Check sheet for the modelled part. Datum: model origin and axes. Units: mm. A direction names the side the tool comes from. Coordinates: 2 decimals unless noted, no trailing zeros. Write each loop counter-clockwise with the first axis right and the second up, starting at its lowest first coordinate (ties: lowest second). Pieces come first, ordered by that corner, then holes. Notation, with made-up numbers: (6.5, -5) -> (40.5, -5) arc R17 cw to (40.5, 2) -> close; hole circle Ø2 at (-39.5, -38.5). An arc over 180 degrees is marked (long way). Put each result on its own line as item: value.
```python
from build123d import *

# Parameters (mm, degrees)
AUFSATZ_LINEAR_AUSTRAGEN1_DEPTH = 18
AUFSATZ_LINEAR_AUSTRAGEN2_DEPTH = 2
SCHNITT_LINEAR_AUSTRAGEN1_REACH = 31.142
SCHNITT_LINEAR_AUSTRAGEN2_REACH = 35.939
SKIZZE5_W                       = 12
SKIZZE5_H                       = 15
SKIZZE7_R                       = 1.22999984
AUFSATZ_LINEAR_AUSTRAGEN3_DEPTH = 6.5
SKIZZE8_R                       = 4.22999984
SKIZZE8_R_2                     = 2.3
AUFSATZ_LINEAR_AUSTRAGEN4_DEPTH = 3
SKIZZE9_W                       = 16.252283896
SKIZZE9_H                       = 8
SKIZZE9_W_2                     = 16.225392475
AUFSATZ_LINEAR_AUSTRAGEN7_DEPTH = 3
SCHNITT_LINEAR_AUSTRAGEN3_REACH = 3.5
SKIZZE11_W                      = 10
SKIZZE11_H                      = 10
SCHNITT_LINEAR_AUSTRAGEN4_REACH = 24.734
SKIZZE13_W                      = 10
SKIZZE13_H                      = 10
SCHNITT_LINEAR_AUSTRAGEN5_REACH = 24.815
SKIZZE14_W                      = 10
SKIZZE14_H                      = 10
SCHNITT_LINEAR_AUSTRAGEN6_REACH = 3.5
SKIZZE15_W                      = 10
SKIZZE15_H                      = 10
SCHNITT_LINEAR_AUSTRAGEN7_REACH = 24.918
SKIZZE16_W                      = 10
SKIZZE16_H                      = 10
SCHNITT_LINEAR_AUSTRAGEN8_REACH = 24.774
SKIZZE17_W                      = 10
SKIZZE17_H                      = 10


with BuildPart() as part:
    # Skizze1 → Aufsatz-Linear austragen1 (new body)
    with BuildSketch(Plane.XY):
        Polygon((-22.149859894, 27.765281808), (-11.635793215, 33.83000044), (-10.65000108, 33.83000044), (-10.65000108, 70.94999986), (10.5900012, 70.94999986), (10.5900012, 33.83000044), (11.612735063, 33.83000044), (21.946878227, 27.90320319), (54.822266278, 46.860690996), (65.431940836, 28.488460753), (35.875483821, 11.41999954), (37.79000014, 11.41999954), (37.79000014, -11.66999904), (36.372671479, -11.66999904), (65.402118422, -28.428154068), (54.791716349, -46.801638497), (21.961456264, -27.849347945), (11.636228403, -33.81000048), (10.608764603, -33.81000048), (10.588764643, -70.99999976), (-10.63000112, -70.99999976), (-10.63000112, -33.81000048), (-11.635211495, -33.81000048), (-21.94526311, -27.869445957), (-54.832668225, -46.841377939), (-65.441180026, -28.458395245), (-33.1799992, -9.82193495), (-33.1799992, 9.582671858), (-65.619428736, 28.349034811), (-55.023633975, 46.732102334), align=None)
        Polygon((-22.149950537, 26.033576659), (-11.234189479, 32.33000044), (-9.15000108, 32.33000044), (-9.15000108, 69.44999986), (9.0900012, 69.44999986), (9.0900012, 32.33000044), (11.2131258, 32.33000044), (21.948913697, 26.172853479), (54.272963006, 44.812413555), (63.382848908, 29.03729054), (31.311020441, 10.516235735), (31.653238716, 9.91999954), (36.29000014, 9.91999954), (36.29000014, -10.16999904), (31.252050971, -10.16999904), (31.132619329, -10.37701429), (63.352910716, -28.977183946), (54.242770108, -44.752743199), (21.961450411, -26.11734559), (11.234340849, -32.31000048), (9.109571053, -32.31000048), (9.089571093, -69.49999976), (-9.13000112, -69.49999976), (-9.13000112, -32.31000048), (-11.233987142, -32.31000048), (-21.945708018, -26.138007916), (-54.2831028, -44.792652518), (-63.392584266, -29.007267794), (-31.162137007, -10.388561496), (-31.6799992, -9.546253935), (-31.6799992, 9.963511331), (-31.471105622, 10.326986156), (-63.571974887, 28.897490395), (-54.473438465, 44.682904625), align=None, mode=Mode.SUBTRACT)
    extrude(amount=AUFSATZ_LINEAR_AUSTRAGEN1_DEPTH)

    # Skizze3 → Aufsatz-Linear austragen2 (add)
    with BuildSketch(Plane(origin=(0, 0, 0), x_dir=(-1, 0, 0), z_dir=(0, 0, -1))):
        Polygon((55.023633975, 46.732102334), (22.149859894, 27.765281808), (11.635793215, 33.83000044), (10.65000108, 33.83000044), (10.65000108, 70.94999986), (-10.5900012, 70.94999986), (-10.5900012, 33.83000044), (-11.612735063, 33.83000044), (-21.946878227, 27.90320319), (-54.822266278, 46.860690996), (-65.431940836, 28.488460753), (-35.875483821, 11.41999954), (-37.79000014, 11.41999954), (-37.79000014, -11.66999904), (-36.372671479, -11.66999904), (-65.402118422, -28.428154068), (-54.791716349, -46.801638497), (-21.961456264, -27.849347945), (-11.636228403, -33.81000048), (-10.608764603, -33.81000048), (-10.588764643, -70.99999976), (10.63000112, -70.99999976), (10.63000112, -33.81000048), (11.635211495, -33.81000048), (21.94526311, -27.869445957), (54.832668225, -46.841377939), (65.441180026, -28.458395245), (33.1799992, -9.82193495), (33.1799992, 9.582671858), (65.619428736, 28.349034811), align=None)
    extrude(amount=AUFSATZ_LINEAR_AUSTRAGEN2_DEPTH)

    # Skizze4 → Schnitt-Linear austragen1 (cut, up to next)
    with BuildSketch(Plane.ZY.offset(-36.29000014), mode=Mode.PRIVATE) as schnitt_linear_austragen1_sk1:
        Polygon((17.00382914, 9.91999954), (17.00382914, -10.16999904), (0.851260669, -10.16999904), (0, -10.16999904), (0, 9.91999954), (0.851260669, 9.91999954), align=None)
    schnitt_linear_austragen1_tool1 = extrude(schnitt_linear_austragen1_sk1.sketch, amount=-SCHNITT_LINEAR_AUSTRAGEN1_REACH, mode=Mode.PRIVATE) & part.part
    add(schnitt_linear_austragen1_tool1.solids().sort_by_distance((36.29, -0.125, 8.501915))[0], mode=Mode.SUBTRACT)

    # Skizze5 → Schnitt-Linear austragen2 (cut, up to next)
    with BuildSketch(Plane(origin=(-31.6799992, 0, 0), x_dir=(0, 0, -1), z_dir=(1, 0, 0)), mode=Mode.PRIVATE) as schnitt_linear_austragen2_sk1:
        with Locations((-6, 0)):
            Rectangle(SKIZZE5_W, SKIZZE5_H)
    schnitt_linear_austragen2_tool1 = extrude(schnitt_linear_austragen2_sk1.sketch, amount=-SCHNITT_LINEAR_AUSTRAGEN2_REACH, mode=Mode.PRIVATE) & part.part
    add(schnitt_linear_austragen2_tool1.solids().sort_by_distance((-31.679999, 0, 6))[0], mode=Mode.SUBTRACT)

    # Skizze7 → Aufsatz-Linear austragen3 (add)
    with BuildSketch(Plane.XY):
        with Locations((0, 15.00000048)):
            Circle(SKIZZE7_R)
        with Locations((0, -18.5000011)):
            Circle(SKIZZE7_R)
        with Locations((-9.1899994, -20.2700001)):
            Circle(SKIZZE7_R)
    extrude(amount=AUFSATZ_LINEAR_AUSTRAGEN3_DEPTH)

    # Skizze8 → Aufsatz-Linear austragen4 (add)
    with BuildSketch(Plane.XY):
        with Locations((-9.1899994, -20.2700001)):
            Circle(SKIZZE8_R)
        with Locations((0, -18.5000011)):
            Circle(SKIZZE8_R)
        with Locations((13.9, 25.897140228)):
            Circle(SKIZZE8_R_2)
        with Locations((-13.9, 25.897140228)):
            Circle(SKIZZE8_R_2)
        with Locations((13.9, -24.8615628)):
            Circle(SKIZZE8_R_2)
        with Locations((-13.9, -24.8615628)):
            Circle(SKIZZE8_R_2)
        with BuildLine():
            Line((3.936452455, 16.548303007), (-3.936452455, 16.548303007))
            ThreePointArc((-3.936452455, 16.548303007), (0, 10.77000064), (3.936452455, 16.548303007))
        make_face()
    extrude(amount=AUFSATZ_LINEAR_AUSTRAGEN4_DEPTH)

    # Skizze9 → Aufsatz-Linear austragen7 (add)
    with BuildSketch(Plane.XY):
        Polygon((-39.106966425, 34.662574989), (-47.255864546, 20.538698219), (-40.326487672, 16.540731718), (-32.177589551, 30.664608488), align=None)
        with Locations((-0.036140748, 47.33000044)):
            Rectangle(SKIZZE9_W, SKIZZE9_H)
        Polygon((40.096213315, 16.744336658), (31.986065924, 30.788205039), (38.913859811, 34.78891396), (47.024007202, 20.745045579), align=None)
        Polygon((40.10078632, -16.697308213), (47.029196881, -20.696949084), (38.916380603, -34.750441337), (31.987970041, -30.750800466), align=None)
        with Locations((-0.017304883, -47.31000048)):
            Rectangle(SKIZZE9_W_2, SKIZZE9_H)
        Polygon((-38.906027405, -34.762365837), (-31.978796823, -30.760681634), (-40.098111463, -16.705508406), (-47.025342045, -20.70719261), align=None)
    extrude(amount=AUFSATZ_LINEAR_AUSTRAGEN7_DEPTH)

    # Skizze11 → Schnitt-Linear austragen3 (cut, up to next)
    with BuildSketch(Plane.XZ.offset(-69.44999986), mode=Mode.PRIVATE) as schnitt_linear_austragen3_sk1:
        with Locations((0, 5)):
            Rectangle(SKIZZE11_W, SKIZZE11_H)
    schnitt_linear_austragen3_tool1 = extrude(schnitt_linear_austragen3_sk1.sketch, amount=-SCHNITT_LINEAR_AUSTRAGEN3_REACH, mode=Mode.PRIVATE) & part.part
    add(schnitt_linear_austragen3_tool1.solids().sort_by_distance((0, 69.45, 5))[0], mode=Mode.SUBTRACT)

    # Skizze13 → Schnitt-Linear austragen4 (cut, up to next)
    with BuildSketch(Plane(origin=(60.106593545, 34.710614216, 0), x_dir=(0, 0, 1), z_dir=(-0.86597514, -0.500087049, 0)), mode=Mode.PRIVATE) as schnitt_linear_austragen4_sk1:
        with Locations((5, 2.556930019)):
            Rectangle(SKIZZE13_W, SKIZZE13_H)
    schnitt_linear_austragen4_tool1 = extrude(schnitt_linear_austragen4_sk1.sketch, amount=-SCHNITT_LINEAR_AUSTRAGEN4_REACH, mode=Mode.PRIVATE) & part.part
    add(schnitt_linear_austragen4_tool1.solids().sort_by_distance((58.827906, 36.924852, 5))[0], mode=Mode.SUBTRACT)

    # Skizze14 → Schnitt-Linear austragen5 (cut, up to next)
    with BuildSketch(Plane(origin=(60.058107222, -34.682624727, 0), x_dir=(0, 0, 1), z_dir=(-0.865975074, 0.500087164, 0)), mode=Mode.PRIVATE) as schnitt_linear_austragen5_sk1:
        with Locations((5, -2.520094297)):
            Rectangle(SKIZZE14_W, SKIZZE14_H)
    schnitt_linear_austragen5_tool1 = extrude(schnitt_linear_austragen5_sk1.sketch, amount=-SCHNITT_LINEAR_AUSTRAGEN5_REACH, mode=Mode.PRIVATE) & part.part
    add(schnitt_linear_austragen5_tool1.solids().sort_by_distance((58.79784, -36.864964, 5))[0], mode=Mode.SUBTRACT)

    # Skizze15 → Schnitt-Linear austragen6 (cut, up to next)
    with BuildSketch(Plane(origin=(0, -69.49999976, 0), x_dir=(1, 0, 0), z_dir=(0, 1, 0)), mode=Mode.PRIVATE) as schnitt_linear_austragen6_sk1:
        with Locations((-0.020215013, -5)):
            Rectangle(SKIZZE15_W, SKIZZE15_H)
    schnitt_linear_austragen6_tool1 = extrude(schnitt_linear_austragen6_sk1.sketch, amount=-SCHNITT_LINEAR_AUSTRAGEN6_REACH, mode=Mode.PRIVATE) & part.part
    add(schnitt_linear_austragen6_tool1.solids().sort_by_distance((-0.020215, -69.5, 5))[0], mode=Mode.SUBTRACT)

    # Skizze16 → Schnitt-Linear austragen7 (cut, up to next)
    with BuildSketch(Plane(origin=(-60.113041463, -34.690230655, 0), x_dir=(0, 0, -1), z_dir=(0.866125522, 0.49982655, 0)), mode=Mode.PRIVATE) as schnitt_linear_austragen7_sk1:
        with Locations((-5, -2.551280899)):
            Rectangle(SKIZZE16_W, SKIZZE16_H)
    schnitt_linear_austragen7_tool1 = extrude(schnitt_linear_austragen7_sk1.sketch, amount=-SCHNITT_LINEAR_AUSTRAGEN7_REACH, mode=Mode.PRIVATE) & part.part
    add(schnitt_linear_austragen7_tool1.solids().sort_by_distance((-58.837844, -36.89996, 5))[0], mode=Mode.SUBTRACT)

    # Skizze17 → Schnitt-Linear austragen8 (cut, up to next)
    with BuildSketch(Plane(origin=(-60.221224503, 34.710841064, 0), x_dir=(0, 0, -1), z_dir=(0.866385869, -0.499375136, 0)), mode=Mode.PRIVATE) as schnitt_linear_austragen8_sk1:
        with Locations((-5, 2.400035044)):
            Rectangle(SKIZZE17_W, SKIZZE17_H)
    schnitt_linear_austragen8_tool1 = extrude(schnitt_linear_austragen8_sk1.sketch, amount=-SCHNITT_LINEAR_AUSTRAGEN8_REACH, mode=Mode.PRIVATE) & part.part
    add(schnitt_linear_austragen8_tool1.solids().sort_by_distance((-59.022707, 36.790198, 5))[0], mode=Mode.SUBTRACT)


solid = part.part
```
Q1. Tool access check on faces 4 (the flat face through (-36, -23.8, 1.5)), 5 (the flat face through (-16.72, -30.88, 8.14)). Record the directions out of +Z, -Z, +X, -X, +Y, -Y that give a thin tool (end or side, any length) a straight path to the whole face; none if there is none.
Recorded:
face 4: +Z
face 5: +Z, -Z, -Y
Q2. Cross-section at A-A (x = -36). Record the cut outline in (y, z), plus the area to 3 significant figures.
Recorded:
outline: (-35.98, -2) -> (-11.45, -2) -> (-11.45, 18) -> (-13.18, 18) -> (-13.18, 0) -> (-23.8, 0) -> (-23.8, 3) -> (-33.08, 3) -> (-33.08, 0) -> (-34.25, 0) -> (-34.25, 18) -> (-35.98, 18) -> close; (11.21, -2) -> (35.76, -2) -> (35.76, 18) -> (34.02, 18) -> (34.02, 0) -> (32.87, 0) -> (32.87, 3) -> (24.04, 3) -> (24.04, 0) -> (12.95, 0) -> (12.95, 18) -> (11.21, 18) -> close
area: 277 mm2
Q3. Material ranges on line 1 along X through (y, z) = (-59, 2.75); line 2 along X through (y, z) = (56.5, 6.75); line 3 along Y through (x, z) = (44.5, 9.5), recorded low to high.
Recorded:
line 1: x = -10.63 to -9.13, 9.1 to 10.6
line 2: x = -10.65 to -9.15, 9.09 to 10.59
line 3: y = -40.86 to -39.13, -18.09 to -16.36, 16.4 to 18.13, 39.18 to 40.91
Q4. Mould release check, pull along Y, two halves, no side actions. Record for faces 1 (the flat face through (16.67, -29.17, 8.87)), 2 (the flat face through (0, -51.31, 1)), 3 (the flat face through (38.61, -37.46, 8.14)): released by +Y, released by -Y, zero draft, split by the parting line, or undercut.
Recorded:
face 1: undercut
face 2: undercut
face 3: released by -Y
Q5. Depth check by flat-ended pin: P1, Ø7.5, axis at x = -36, y = 22.5, coming from the +Z side; P2, Ø1.2, axis at y = -70.5, z = 7.5, coming from the +X side; P3, Ø3, axis at y = 39, z = 15.5, coming from the -X side. Enter the tip coordinate at first touch or a pass-through.
Recorded:
P1: stops at z = 3
P2: stops at x = 10.59
P3: stops at x = -60.34
Q6. Cross-section at B-B (x = 13.9). Record the cut outline in (y, z).
Recorded:
outline: (-32.5, -2) -> (32.52, -2) -> (32.52, 18) -> (30.79, 18) -> (30.79, 0) -> (28.2, 0) -> (28.2, 3) -> (23.6, 3) -> (23.6, 0) -> (-22.56, 0) -> (-22.56, 3) -> (-27.16, 3) -> (-27.16, 0) -> (-30.77, 0) -> (-30.77, 18) -> (-32.5, 18) -> close
